The listing builds one solid part. Answer for the finished solid, in the listing's coordinates (mm). Coordinates: 2 decimals unless noted, no trailing zeros. Order: outer loops, then holes, each group sorted by start corner. A loop starts at its lowest first (then second) coordinate and runs counter-clockwise, first axis right, second up.
```python
from build123d import *

# Parameters (mm, degrees)
BOSS_EXTRU_1_DEPTH      = 10
ESQUISSE2_R             = 2.5
ENL_V_MAT_EXTRU_1_DEPTH = 10


with BuildPart() as part:
    # Esquisse1 → Boss.-Extru.1 (new body)
    with BuildSketch(Plane(origin=(0, 0, 0), x_dir=(1, 0, 0), z_dir=(0, 1, 0))):
        with BuildLine():
            ThreePointArc((-0.943707896, 213.69893991), (3.70122741, 221.970757316), (-4.978017186, 218.140731151))
            ThreePointArc((-4.978017186, 218.140731151), (-59.227468872, 93.60907386), (-4.978017186, -30.92258343))
            ThreePointArc((-4.978017186, -30.92258343), (3.70122741, -34.752609595), (-0.943707895, -26.48079219))
            ThreePointArc((-0.943707895, -26.48079219), (-53.227468872, 93.60907386), (-0.943707896, 213.69893991))
        make_face()
    extrude(amount=BOSS_EXTRU_1_DEPTH)

    # Esquisse2 → Enlèv. mat.-Extru.1 (cut)
    with BuildSketch(Plane(origin=(0, 10, 0), x_dir=(1, 0, 0), z_dir=(0, 1, 0))):
        with Locations(Location((0, 218.60907386, 0), (0, 0, 270))):
            Circle(ESQUISSE2_R)
        with Locations(Location((0, -31.39092614, 0), (0, 0, 270))):
            Circle(ESQUISSE2_R)
    extrude(amount=-ENL_V_MAT_EXTRU_1_DEPTH, mode=Mode.SUBTRACT)


solid = part.part
```
1) A cutting plane is placed at D-D, the plane z = -39.5. Write down the section's boundary in (x, y), plus the area to 3 significant figures.
2) A cutting plane is placed at B-B, the plane x = -19.5. Write down the section's boundary in (y, z), plus the area to 3 significant figures.
3) The mould has two halves that part along Z. Classify faces 1 (the flat face through (-53.4, 0, -94.2)), 2 (the cylindrical face through (-59.216, 4.93, -95.565)), 3 (the cylindrical face through (0.751, 5.07, -216.225)): released by +Z, released by -Z, zero draft, split by the parting line, or undercut.
4) A cutting plane is placed at A-A, the plane y = 6.25. Write down the section's boundary in (x, z).
5) Each of these flat-tipped pins is pushed along its axis until it touches: P1, Ø5, axis at x = -4, y = 5.5, coming from the +Z side; P2, Ø4, axis at x = -21, y = 4, coming from the +Z side; P3, Ø1, axis at x = -20.5, y = 2, coming from the +Z side. Where does it stop, or does it pass through?
6) A cutting plane is placed at C-C, the plane x = -50. Write down the section's boundary in (y, z), plus the area to 3 significant figures.
7) Straight lines are drawn through the part: probe 1 along Z at (x, y) = (-1.5, 2.75); probe 2 along Z at (x, y) = (-19, 3.25); probe 3 along Z at (x, y) = (-20.5, 3.25). For each, find the intervals that lie inside material, in ascending order.
Working result:
1. outline: (-50.39, 0) - (-44.05, 0) - (-44.05, 10) - (-50.39, 10) - close
1. area: 63.4 mm2
2. outline: (0, -202.85) - (10, -202.85) - (10, -193.25) - (0, -193.25) - close; (0, 6.04) - (10, 6.04) - (10, 15.63) - (0, 15.63) - close
2. area: 192 mm2
3. face 1: zero draft
3. face 2: split by the parting line
3. face 3: undercut
4. outline: (-4.98, -218.14) arc R5 ccw (long way) to (-0.94, -213.7) arc R164.06 cw to (-0.94, 26.48) arc R5 ccw (long way) to (-4.98, 30.92) arc R170.06 ccw to start; hole circle Ø5 at (0, -218.61); hole circle Ø5 at (0, 31.39)
5. P1: stops at z = 36.16
5. P2: stops at z = 16.23
5. P3: stops at z = 15.03
6. outline: (0, -148.87) - (10, -148.87) - (10, -125.99) - (0, -125.99) - close; (0, -61.23) - (10, -61.23) - (10, -38.35) - (0, -38.35) - close
6. area: 457 mm2
7. probe 1: z = -223.38 to -220.61, -216.61 to -213.18, 25.96 to 29.39, 33.39 to 36.16
7. probe 2: z = -203.44 to -193.9, 6.69 to 16.23
7. probe 3: z = -201.65 to -191.93, 4.71 to 14.43
